Geometry check sheet. Reference: the model listing, model coordinates, mm. A direction names the side the tool comes from. Coordinates: 2 decimals unless noted, no trailing zeros. Write each loop counter-clockwise with the first axis right and the second up, starting at its lowest first coordinate (ties: lowest second). Pieces come first, ordered by that corner, then holes. Notation, with made-up numbers: M -9,10 L 15,10 A17 ccw 15,21 Z; hole C 20,79.25 d4. An arc over 180 degrees is marked long. Write each question's results on one line, items separated by ' | '.
```python
from build123d import *

# Parameters (mm, degrees)
CROQUIS2_W              = 39.5
CROQUIS2_H              = 47.5
CROQUIS2_R              = 2.1
SALIENTE_EXTRUIR1_DEPTH = 5
REDONDEO1_R             = 4
CROQUIS3_R              = 4.05
CORTAR_EXTRUIR1_DEPTH   = 2.8


with BuildPart() as part:
    # Croquis2 → Saliente-Extruir1 (new body)
    with BuildSketch(Plane.XY):
        with Locations((19.75, 23.75)):
            Rectangle(CROQUIS2_W, CROQUIS2_H)
        with Locations((9.75, 10)):
            Circle(CROQUIS2_R, mode=Mode.SUBTRACT)
        with Locations((29.75, 10)):
            Circle(CROQUIS2_R, mode=Mode.SUBTRACT)
        with BuildLine():
            Line((12.4, 41.171297972), (12.4, 33.911297972))
            ThreePointArc((12.4, 33.911297972), (9.75, 31.261297972), (7.1, 33.911297972))
            Line((7.1, 33.911297972), (7.1, 41.171297972))
            ThreePointArc((7.1, 41.171297972), (9.75, 43.821297972), (12.4, 41.171297972))
        make_face(mode=Mode.SUBTRACT)
        with BuildLine():
            Line((22.4, 41.171297972), (22.4, 33.911297972))
            ThreePointArc((22.4, 33.911297972), (19.75, 31.261297972), (17.1, 33.911297972))
            Line((17.1, 33.911297972), (17.1, 41.171297972))
            ThreePointArc((17.1, 41.171297972), (19.75, 43.821297972), (22.4, 41.171297972))
        make_face(mode=Mode.SUBTRACT)
        with BuildLine():
            Line((32.4, 41.171297972), (32.4, 33.911297972))
            ThreePointArc((32.4, 33.911297972), (29.75, 31.261297972), (27.1, 33.911297972))
            Line((27.1, 33.911297972), (27.1, 41.171297972))
            ThreePointArc((27.1, 41.171297972), (29.75, 43.821297972), (32.4, 41.171297972))
        make_face(mode=Mode.SUBTRACT)
    extrude(amount=SALIENTE_EXTRUIR1_DEPTH)

    # Redondeo1
    redondeo1_edges = [part.edges().sort_by_distance(p)[0] for p in [
        (0, 47.5, 2.5),
        (39.5, 47.5, 2.5),
        (39.5, 0, 2.5),
        (0, 0, 2.5),
    ]]
    fillet(redondeo1_edges, radius=REDONDEO1_R)

    # Croquis3 → Cortar-Extruir1 (cut)
    with BuildSketch(Plane.XY.offset(5)):
        with Locations((29.75, 10)):
            Circle(CROQUIS3_R)
        with Locations((9.75, 10)):
            Circle(CROQUIS3_R)
    extrude(amount=-CORTAR_EXTRUIR1_DEPTH, mode=Mode.SUBTRACT)


solid = part.part
```
Q1. Sectioned sample at D-D on x = 9.75. Record the cut outline in (y, z).
Geometry check:
outline: M 0,0 L 7.9,0 L 7.9,2.2 L 5.95,2.2 L 5.95,5 L 0,5 Z; M 12.1,0 L 31.26,0 L 31.26,5 L 14.05,5 L 14.05,2.2 L 12.1,2.2 Z; M 43.82,0 L 47.5,0 L 47.5,5 L 43.82,5 Z
Q2. Sectioned sample at B-B on z = 1.3. Record the cut outline in (x, y), and give its area (3 significant figures).
Geometry check:
outline: M 0,4 A4 ccw 4,0 L 35.5,0 A4 ccw 39.5,4 L 39.5,43.5 A4 ccw 35.5,47.5 L 4,47.5 A4 ccw 0,43.5 Z; hole M 7.1,33.91 A2.65 ccw 12.4,33.91 L 12.4,41.17 A2.65 ccw 7.1,41.17 Z; hole C 9.75,10 d4.2; hole M 17.1,33.91 A2.65 ccw 22.4,33.91 L 22.4,41.17 A2.65 ccw 17.1,41.17 Z; hole M 27.1,33.91 A2.65 ccw 32.4,33.91 L 32.4,41.17 A2.65 ccw 27.1,41.17 Z; hole C 29.75,10 d4.2 | area: 1,650 mm2
Q3. Mould release check, pull along Y, two halves, no side actions. Record for faces 4 (the cylindrical face through (38.297, 1.141, 2.535)), 5 (the flat face through (20, 47.5, 2)), 6 (the flat face through (32.4, 38, 2)): pulls with the +Y half, pulls with the -Y half, needs draft (parallel to the pull), parting line crosses it, or undercut.
Geometry check:
face 4: pulls with the -Y half | face 5: pulls with the +Y half | face 6: undercut
Q4. Depth check by flat-ended pin: P1, Ø6.5, axis at x = 9, y = 10.5, coming from the +Z side. Enter the tip coordinate at first touch or a pass-through.
Geometry check:
P1: stops at z = 5
Q5. Sectioned sample at A-A on y = 37.5. Record the cut outline in (x, z).
Geometry check:
outline: M 0,0 L 7.1,0 L 7.1,5 L 0,5 Z; M 12.4,0 L 17.1,0 L 17.1,5 L 12.4,5 Z; M 22.4,0 L 27.1,0 L 27.1,5 L 22.4,5 Z; M 32.4,0 L 39.5,0 L 39.5,5 L 32.4,5 Z
Q6. Access from +Z, -Z, +X, -X, +Y, -Y to the whole of each face (thin tool, end or side, straight path). Record for faces 1 (the cylindrical face through (29.81, 31.26, 2.46)), 2 (the flat face through (0, 23, 2)), 3 (the cylindrical face through (33.61, 11.22, 3.62)).
Geometry check:
face 1: +Z, -Z | face 2: +Z, -Z, -X, +Y, -Y | face 3: +Z
Q7. Scan lines: probe 1 along X at (y, z) = (10, 1.15); probe 2 along X at (y, z) = (40, 3.9); probe 3 along Y at (x, z) = (29.75, 1.75). Record each from-to range of solid material in increasing order.
Geometry check:
probe 1: x = 0 to 7.65, 11.85 to 27.65, 31.85 to 39.5 | probe 2: x = 0 to 7.1, 12.4 to 17.1, 22.4 to 27.1, 32.4 to 39.5 | probe 3: y = 0 to 7.9, 12.1 to 31.26, 43.82 to 47.5
Q8. Sectioned sample at C-C on x = 19.75. Record the cut outline in (y, z).
Geometry check:
outline: M 0,0 L 31.26,0 L 31.26,5 L 0,5 Z; M 43.82,0 L 47.5,0 L 47.5,5 L 43.82,5 Z
